```python
from build123d import *

# Parameters (mm, degrees)
SKETCH1_R           = 2.1209
BOSS_EXTRUDE1_DEPTH = 6.35


with BuildPart() as part:
    # Sketch1 → Boss-Extrude1 (new body)
    # profile 1 of 3: a face of its own
    with BuildSketch(Plane(origin=(0, 0, 0), x_dir=(1, 0, 0), z_dir=(0, 1, 0))):
        with BuildLine():
            ThreePointArc((132.08, -74.295), (137.317671124, -104.024937773), (152.4, -130.175))
            Line((152.4, -130.175), (152.4, 0))
            Line((152.4, 0), (12.7, 0))
            Line((12.7, 0), (12.7, -109.900328253))
            ThreePointArc((12.7, -109.900328253), (18.3936727, -92.500794407), (20.32, -74.295))
            ThreePointArc((20.32, -74.295), (76.2, -18.415), (132.08, -74.295))
        make_face()
        with Locations(Location((19.05, -44.45, 0), (0, 0, 270))):
            Circle(SKETCH1_R, mode=Mode.SUBTRACT)
        with Locations(Location((19.05, -6.35, 0), (0, 0, 270))):
            Circle(SKETCH1_R, mode=Mode.SUBTRACT)
    # profile 2 of 3: a face of its own
    with BuildSketch(Plane(origin=(0, 0, 0), x_dir=(1, 0, 0), z_dir=(0, 1, 0))):
        with BuildLine():
            Line((152.4, 0), (152.4, -130.175))
            ThreePointArc((152.4, -130.175), (167.482328876, -104.024937773), (172.72, -74.295))
            ThreePointArc((172.72, -74.295), (228.6, -18.415), (284.48, -74.295))
            ThreePointArc((284.48, -74.295), (289.717671124, -104.024937773), (304.8, -130.175))
            Line((304.8, -130.175), (304.8, 0))
            Line((304.8, 0), (152.4, 0))
        make_face()
    # profile 3 of 3: a face of its own
    with BuildSketch(Plane(origin=(0, 0, 0), x_dir=(1, 0, 0), z_dir=(0, 1, 0))):
        with BuildLine():
            Line((444.5, 0), (304.8, 0))
            Line((304.8, 0), (304.8, -130.175))
            ThreePointArc((304.8, -130.175), (319.882328876, -104.024937773), (325.12, -74.295))
            ThreePointArc((325.12, -74.295), (381, -18.415), (436.88, -74.295))
            ThreePointArc((436.88, -74.295), (438.8063273, -92.500794407), (444.5, -109.900328253))
            Line((444.5, -109.900328253), (444.5, 0))
        make_face()
        with Locations(Location((438.15, -44.45, 0), (0, 0, 270))):
            Circle(SKETCH1_R, mode=Mode.SUBTRACT)
        with Locations(Location((438.15, -6.35, 0), (0, 0, 270))):
            Circle(SKETCH1_R, mode=Mode.SUBTRACT)
    extrude(amount=-BOSS_EXTRUDE1_DEPTH)


solid = part.part
```
Input: part model. Units: mm. Frame: model coordinates. A direction names the side the tool comes from. Round coordinates to 2 decimals unless told otherwise and drop trailing zeros. Loops run counter-clockwise (first coordinate to the right, second up) from the corner with the lowest first, then second, coordinate; pieces in that order, holes last. Notation, with made-up numbers: (-20.75, -27.5) - (0.25, -27.5) arc R7 cw to (0.25, -16.5) - close; hole circle Ø5 at (47, 59.5). An arc over 180 degrees is marked (long way). One line per item, written item: value. Start each with the question number.
(1) Access query for faces 1 (the cylindrical face through (289.573, -3.131, 103.625)), 2 (the flat face through (228, -6.35, 17)). Directions: +Z, -Z, +X, -X, +Y, -Y. A direction counts if a zero-diameter tool reaches every point of the face in a straight line with its end or side. Return the directions, or none.
(2) Section A-A, the plane y = -4.25. Return loops of the section in (x, z) (3 decimals), plus the area to 3 significant figures.
(3) Contact query for flat-ended pins moving along their axis: P1, Ø2.5, axis at x = 438.15, z = 6.35, coming from the +Y side; P2, Ø5, axis at x = 19.05, z = 44.45, coming from the -Y side. Output: stop coordinate, or through.
(4) Section C-C, the plane x = 381. Return loops of the section in (y, z) (3 decimals), plus the area to 3 significant figures.
(5) Ray query, line 1 (X direction, y = -1.5, z = 6.35); line 2 (X direction, y = -1.25, z = 29.5); line 3 (X direction, y = -2.5, z = 74.5). Return the intervals inside material, ascending. Write a range as [from, to].
(6) Section D-D, the plane z = 30. Return loops of the section in (x, y).
(7) Section B-B, the plane z = 80.5. Return loops of the section in (x, y), plus the area to 3 significant figures.
Results below:
1. face 1: +Z, +Y, -Y
1. face 2: +Z, -Z, +X, -X, -Y
2. outline: (12.7, 0) - (444.5, 0) - (444.5, 109.9) arc R86.995 ccw to (436.88, 74.295) arc R55.88 cw to (325.12, 74.295) arc R86.995 ccw to (304.8, 130.175) arc R86.995 ccw to (284.48, 74.295) arc R55.88 cw to (172.72, 74.295) arc R86.995 ccw to (152.4, 130.175) arc R86.995 ccw to (132.08, 74.295) arc R55.88 cw to (20.32, 74.295) arc R86.995 ccw to (12.7, 109.9) - close; hole circle Ø4.242 at (19.05, 6.35); hole circle Ø4.242 at (19.05, 44.45); hole circle Ø4.242 at (438.15, 6.35); hole circle Ø4.242 at (438.15, 44.45)
2. area: 20,800 mm^2
3. P1: through
3. P2: y = -6.35
4. outline: (-6.35, 0) - (0, 0) - (0, 18.415) - (-6.35, 18.415) - close
4. area: 117 mm^2
5. line 1: [12.7, 16.93], [21.17, 436.03], [440.27, 444.5]
5. line 2: [12.7, 42.79], [109.61, 195.19], [262.01, 347.59], [414.41, 444.5]
5. line 3: [12.7, 20.32], [132.08, 172.72], [284.48, 325.12], [436.88, 444.5]
6. outline: (12.7, -6.35) - (42.13, -6.35) - (42.13, 0) - (12.7, 0) - close; (110.27, -6.35) - (194.53, -6.35) - (194.53, 0) - (110.27, 0) - close; (262.67, -6.35) - (346.93, -6.35) - (346.93, 0) - (262.67, 0) - close; (415.07, -6.35) - (444.5, -6.35) - (444.5, 0) - (415.07, 0) - close
7. outline: (12.7, -6.35) - (20.1, -6.35) - (20.1, 0) - (12.7, 0) - close; (132.3, -6.35) - (172.5, -6.35) - (172.5, 0) - (132.3, 0) - close; (284.7, -6.35) - (324.9, -6.35) - (324.9, 0) - (284.7, 0) - close; (437.1, -6.35) - (444.5, -6.35) - (444.5, 0) - (437.1, 0) - close
7. area: 604 mm^2
